Can you work these out from the model? Positions are in its coordinate system, mm. A direction names the side the tool comes from. Give positions to 0.01 mm unless a question says otherwise; leave off trailing zeros. Use a Markdown table: item, result. Add a question column.
from build123d import *

# Parameters (mm, degrees)
BOSS_EXTRU_1_DEPTH           = 5
BOSS_EXTRU_2_DEPTH           = 5
BOSS_EXTRU_2_DEPTH_BACK      = 5
BOSS_EXTRU_3_DEPTH           = 5
BOSS_EXTRU_3_DEPTH_BACK      = 5
ESQUISSE7_R                  = 2
ENL_V_MAT_EXTRU_4_DEPTH      = 225.666419389
ENL_V_MAT_EXTRU_4_DEPTH_BACK = 225.666419389
ENL_V_MAT_EXTRU_6_DEPTH      = 225.666419389
ENL_V_MAT_EXTRU_6_DEPTH_BACK = 225.666419389
CHANFREIN1_SIZE              = 0.5


with BuildPart() as part:
    # Esquisse1 → Boss.-Extru.1 (new body)
    with BuildSketch(Plane.XY):
        with BuildLine():
            Line((-120.208152802, 115.814760073), (120.208152802, 115.814760073))
            Line((120.208152802, 115.814760073), (120.208152802, 120.208152802))
            ThreePointArc((120.208152802, 120.208152802), (0, 170), (-120.208152802, 120.208152802))
            Line((-120.208152802, 120.208152802), (-120.208152802, 115.814760073))
        make_face()
    extrude(amount=BOSS_EXTRU_1_DEPTH)

    # Esquisse2 → Boss.-Extru.2 (add, two sides: drawn at the far end of the back side and taken through both)
    with BuildSketch(Plane(origin=(0, 0, 0), x_dir=(-1, 0, 0), z_dir=(0, 0, -1)).offset(-BOSS_EXTRU_2_DEPTH_BACK)):
        with BuildLine():
            Line((127.279220614, 127.279220614), (120.208152802, 120.208152802))
            ThreePointArc((120.208152802, 120.208152802), (0, 170), (-120.208152802, 120.208152802))
            Line((-120.208152802, 120.208152802), (-127.279220614, 127.279220614))
            ThreePointArc((-127.279220614, 127.279220614), (0, 180), (127.279220614, 127.279220614))
        make_face()
    extrude(amount=BOSS_EXTRU_2_DEPTH + BOSS_EXTRU_2_DEPTH_BACK)

    # Enlèvement de matière-Balayage1: sweep along a path in Esquisse3
    with BuildLine(Plane(origin=(0, 0, 0), x_dir=(-1, 0, 0), z_dir=(0, 0, -1))) as enl_vement_de_mati_re_balayage1_path:
        ThreePointArc((126.572113832, 126.572113832), (0, 179), (-126.572113832, 126.572113832))
    # Esquisse5 → Enlèvement de matière-Balayage1 (sweep, cut)
    with BuildSketch(Plane(origin=(0, 0, 0), x_dir=(0, 0, -1), z_dir=(0.7071067811865468, -0.7071067811865483, 0))):
        with BuildLine():
            Line((-0.939692621, 176.657979857), (-2.156088475, 180))
            Line((-2.156088475, 180), (2.156088475, 180))
            Line((2.156088475, 180), (0.939692621, 176.657979857))
            ThreePointArc((0.939692621, 176.657979857), (0, 176), (-0.939692621, 176.657979857))
        make_face()
    sweep(path=enl_vement_de_mati_re_balayage1_path.line, mode=Mode.SUBTRACT)

    # Esquisse7 → Boss.-Extru.3 (add, two sides: drawn at the far end of the back side and taken through both)
    with BuildSketch(Plane(origin=(0, 0, 0), x_dir=(-1, 0, 0), z_dir=(0, 0, -1)).offset(-BOSS_EXTRU_3_DEPTH_BACK)):
        Polygon((-123.743686708, 123.743686708), (-134.350288425, 134.350288425), (-127.279220614, 141.421356237), (-116.672618896, 130.81475452), align=None)
        with Locations((-125.511453661, 132.582521472)):
            Circle(ESQUISSE7_R, mode=Mode.SUBTRACT)
    extrude(amount=BOSS_EXTRU_3_DEPTH + BOSS_EXTRU_3_DEPTH_BACK)

    # Esquisse8 → Enlèv. mat.-Extru.4 (cut, two sides: drawn at the far end of the back side and taken through both)
    with BuildSketch(Plane(origin=(0, 0, 0), x_dir=(-1, 0, 0), z_dir=(0, 0, -1)).offset(-ENL_V_MAT_EXTRU_4_DEPTH_BACK)):
        Polygon((-120.208152802, 120.208152802), (-104.630387374, 104.630387374), (-145.023097607, 109.535343621), (-125.124551125, 125.124551125), align=None)
        Polygon((127.279220614, 127.279220614), (100.741517302, 100.741517302), (140.507843055, 93.246561367), align=None)
    extrude(amount=ENL_V_MAT_EXTRU_4_DEPTH + ENL_V_MAT_EXTRU_4_DEPTH_BACK, mode=Mode.SUBTRACT)

    # Esquisse10 → Enlèv. mat.-Extru.6 (cut, two sides: drawn at the far end of the back side and taken through both)
    with BuildSketch(Plane(origin=(0, 0, 0), x_dir=(-1, 0, 0), z_dir=(0, 0, -1)).offset(-ENL_V_MAT_EXTRU_6_DEPTH_BACK)):
        with BuildLine():
            Line((-25.791169082, 149.314760073), (-15.791169082, 149.314760073))
            ThreePointArc((-15.791169082, 149.314760073), (-13.291169082, 146.814760073), (-15.791169082, 144.314760073))
            Line((-15.791169082, 144.314760073), (-25.791169082, 144.314760073))
            ThreePointArc((-25.791169082, 144.314760073), (-28.291169082, 146.814760073), (-25.791169082, 149.314760073))
        make_face()
        with BuildLine():
            Line((-25.791169082, 130.314760073), (-15.791169082, 130.314760073))
            ThreePointArc((-15.791169082, 130.314760073), (-13.291169082, 127.814760073), (-15.791169082, 125.314760073))
            Line((-15.791169082, 125.314760073), (-25.791169082, 125.314760073))
            ThreePointArc((-25.791169082, 125.314760073), (-28.291169082, 127.814760073), (-25.791169082, 130.314760073))
        make_face()
    extrude(amount=ENL_V_MAT_EXTRU_6_DEPTH + ENL_V_MAT_EXTRU_6_DEPTH_BACK, mode=Mode.SUBTRACT)

    # Chanfrein1
    chanfrein1_edges = [part.edges().sort_by_distance(p)[0] for p in [
        (0, 115.814760073, 0),
    ]]
    chamfer(chanfrein1_edges, length=CHANFREIN1_SIZE)


solid = part.part
1. We'd pull the mould along X, two halves only. Please class faces 6 (the face through (2.9, 170.2, -5)), 7 (the face through (130.9, 137.8, 0.1)), 8 (the face through (28.29, 146.76, 2.53)): +X half, -X half, draft (parallel to the pull), parting line (faces both ways), or undercut.
2. On a 3-axis mill with a long thin cutter (end or side, diameter ignored), from which of +Z, -Z, +X, -X, +Y, -Y can I reach the whole of each face in a straight line? I mean faces 1 (the face through (-2, 138, 0)), 2 (the face through (21, 125.315, 3)), 3 (the face through (-3.093, 179.973, -3.558)), 4 (the face through (-6.79, 176.737, -1.016)), 5 (the face through (-2, 115.815, 3)). Say none if no direction works.
3. I need wall thicknesses on L1, parallel to Z at x = -101.5, y = 131; L2, parallel to X at y = 142, z = -4.5; L3, parallel to X at y = 147.5, z = -0.25. Which ranges of each line are inside material? Lowest first, please. Write a range as [from, to].
4. Will these pins go through, and if not, where does the flat tip stop? pin 1 (3 mm diameter, centred on x = 125.51, y = 132.58, fed in from -Z); pin 2 (1 mm diameter, centred on x = 75, z = -2, fed in from -Y); pin 3 (4 mm diameter, centred on x = 20.5, z = 3, fed in from +Y); pin 4 (4 mm diameter, centred on y = 158.5, z = -3, fed in from -X).
Geometry results:
| question | item | result |
|---|---|---|
| 1 | face 6 | draft |
| 1 | face 7 | +X half |
| 1 | face 8 | undercut |
| 2 | face 1 | -Z, -Y |
| 2 | face 2 | +Z, -Z |
| 2 | face 3 | +Z, -Z, +Y |
| 2 | face 4 | +Y |
| 2 | face 5 | +Z, -Z, +X, -X, -Y |
| 3 | L1 | z = [0, 5] |
| 3 | L2 | x = [-110.62, -93.47], [93.47, 110.62] |
| 3 | L3 | x = [-96.08, -84.52], [84.52, 96.08] |
| 4 | pin 1 | passes through |
| 4 | pin 2 | stops at y = 152.31 |
| 4 | pin 3 | stops at y = 179.05 |
| 4 | pin 4 | stops at x = -88.93 |
